Study the drawing (mm; zero at the part's minimum x, y, z) and answer. Give positions to 0.01 mm unless a question says otherwise; leave off trailing zeros. Order: outer loops, then holes, each group sorted by start corner. A loop starts at its lowest first (then second) coordinate and runs counter-clockwise, first axis right, second up. Notation, with made-up numbers: (46.25, -11.5) - (51.25, -11.5) arc R23 ccw to (51.25, 5.5) - close; hole circle Ø2 at (24, -31.5). An arc over 180 degrees is marked (long way). Put each result on its own line as item: value.
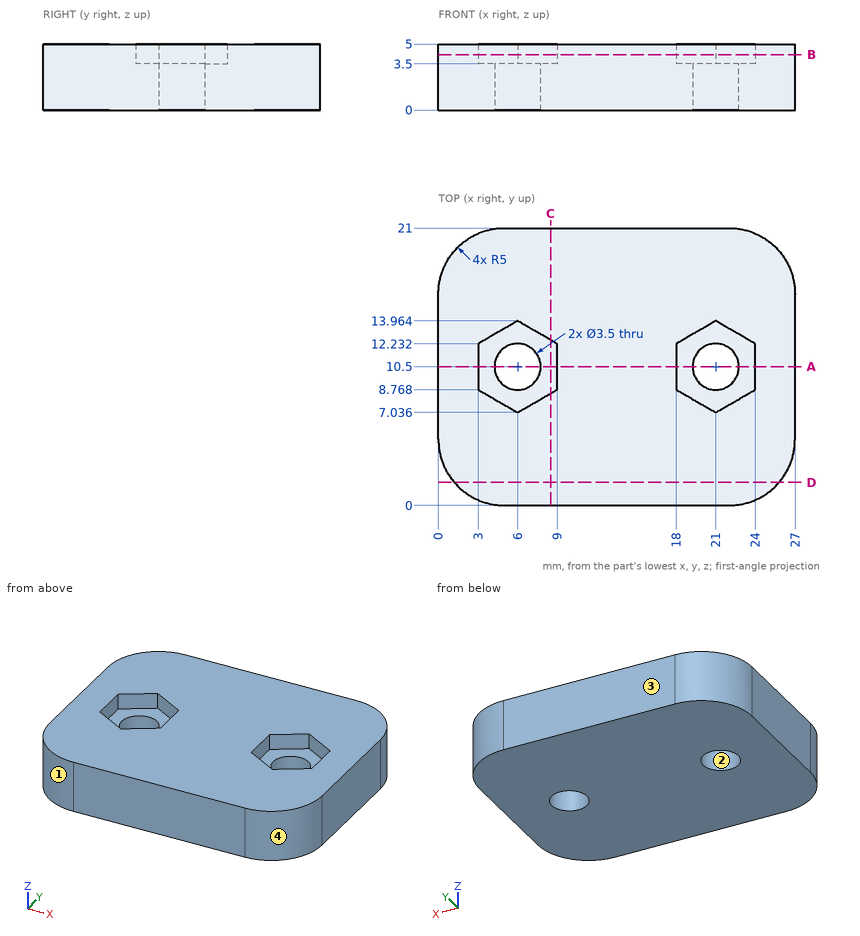
(1) Straight lines are drawn through the part: line 1 (Y direction, x = 21, z = 1.9); line 2 (X direction, y = 7.5, z = 4.2); line 3 (X direction, y = 10, z = 1.2). For each, find the intervals that lie inside material, in ascending order.
Geometry check:
line 1: y = 0 to 8.75, 12.25 to 21
line 2: x = 0 to 5.2, 6.8 to 20.2, 21.8 to 27
line 3: x = 0 to 4.32, 7.68 to 19.32, 22.68 to 27
(2) Section A-A, the plane y = 10.5 is taken. Write down the section's boundary in (x, z), then the cut area to 3 significant figures.
Geometry check:
outline: (0, 0) - (4.25, 0) - (4.25, 3.5) - (3, 3.5) - (3, 5) - (0, 5) - close; (7.75, 0) - (19.25, 0) - (19.25, 3.5) - (18, 3.5) - (18, 5) - (9, 5) - (9, 3.5) - (7.75, 3.5) - close; (22.75, 0) - (27, 0) - (27, 5) - (24, 5) - (24, 3.5) - (22.75, 3.5) - close
area: 92.5 mm²
(3) Section D-D, the plane y = 1.75 is taken. Write down the section's boundary in (x, z).
Geometry check:
outline: (1.2, 0) - (25.8, 0) - (25.8, 5) - (1.2, 5) - close
(4) Determine the mould class of the marked faces 1, 2, 3 and 4 for opening direction X: pulls with the +X half, pulls with the -X half, needs draft (parallel to the pull), parting line crosses it, or undercut.
Geometry check:
face 1: pulls with the -X half
face 2: undercut
face 3: needs draft
face 4: pulls with the +X half
(5) Section B-B, the plane z = 4.2 is taken. Write down the section's boundary in (x, y).
Geometry check:
outline: (0, 5) arc R5 ccw to (5, 0) - (22, 0) arc R5 ccw to (27, 5) - (27, 16) arc R5 ccw to (22, 21) - (5, 21) arc R5 ccw to (0, 16) - close; hole (3, 8.77) - (6, 7.04) - (9, 8.77) - (9, 12.23) - (6, 13.96) - (3, 12.23) - close; hole (18, 8.77) - (21, 7.04) - (24, 8.77) - (24, 12.23) - (21, 13.96) - (18, 12.23) - close
(6) Section C-C, the plane x = 8.5 is taken. Write down the section's boundary in (y, z).
Geometry check:
outline: (0, 0) - (21, 0) - (21, 5) - (12.52, 5) - (12.52, 3.5) - (8.48, 3.5) - (8.48, 5) - (0, 5) - close
(7) Given pin 1 (3 mm diameter, centred on x = 6, y = 9.5, fed in from +Z); pin 2 (2 mm diameter, centred on x = 6, y = 10.5, fed in from -Z), each flat-ended and moving along its own axis, determine where each tip first touches the part or whether it passes through.
Geometry check:
pin 1: stops at z = 3.5
pin 2: passes through
